Source: CAD feature listing. Evaluate the final solid. Frame: model axes, mm. Face numbers are marked on the shaded views. Give positions to 0.01 mm unless a question says otherwise; leave off trailing zeros. Write item = value, one per line.
from build123d import *

# Parameters (mm, degrees)
SKETCH_1_R          = 15
SKETCH_1_R_2        = 1.45
SKETCH_1_R_3        = 1.5
EXTRUDE_1_DEPTH     = 8
SKETCH_2_R          = 1.45
SKETCH_2_R_2        = 1.5
EXTRUDE_2_DEPTH     = 7
SKETCH_3_R          = 1.45
CUT_EXTRUDE_1_DEPTH = 8
SKETCH_4_R          = 1.45
CUT_EXTRUDE_2_DEPTH = 8
SKETCH_5_R          = 1.45
CUT_EXTRUDE_3_DEPTH = 8
SKETCH_6_R          = 1.45
CUT_EXTRUDE_4_DEPTH = 8
SKETCH_7_R          = 1.45
CUT_EXTRUDE_5_DEPTH = 8
SKETCH_8_R          = 1.5
CUT_EXTRUDE_6_DEPTH = 8
CHAMFER_1_SIZE      = 1.55


with BuildPart() as part:
    # 草图1 → 凸台-拉伸1 (new body)
    with BuildSketch(Plane(origin=(0, 0, 0), x_dir=(1, 0, 0), z_dir=(0, 1, 0))):
        Circle(SKETCH_1_R)
        with Locations((0, 12)):
            Circle(SKETCH_1_R_2, mode=Mode.SUBTRACT)
        with Locations((-10.392304845, -6)):
            Circle(SKETCH_1_R_2, mode=Mode.SUBTRACT)
        with Locations((10.392304845, -6)):
            Circle(SKETCH_1_R_2, mode=Mode.SUBTRACT)
        with Locations((-11.258330249, 6.5)):
            Circle(SKETCH_1_R_3, mode=Mode.SUBTRACT)
        with Locations((0, -13)):
            Circle(SKETCH_1_R_3, mode=Mode.SUBTRACT)
        with Locations((11.258330249, 6.5)):
            Circle(SKETCH_1_R_3, mode=Mode.SUBTRACT)
    extrude(amount=EXTRUDE_1_DEPTH)

    # 草图2 → 凸台-拉伸2 (add)
    with BuildSketch(Plane(origin=(0, 8, 0), x_dir=(1, 0, 0), z_dir=(0, 1, 0))):
        Polygon((0, 17.320508076), (-15, 8.660254038), (-15, -8.660254038), (0, -17.320508076), (15, -8.660254038), (15, 8.660254038), align=None)
        with Locations((0, 12)):
            Circle(SKETCH_2_R, mode=Mode.SUBTRACT)
        with Locations((-11.258330249, 6.5)):
            Circle(SKETCH_2_R_2, mode=Mode.SUBTRACT)
        with Locations((11.258330249, 6.5)):
            Circle(SKETCH_2_R_2, mode=Mode.SUBTRACT)
        with Locations((-10.392304845, -6)):
            Circle(SKETCH_2_R, mode=Mode.SUBTRACT)
        with Locations((0, -13)):
            Circle(SKETCH_2_R_2, mode=Mode.SUBTRACT)
        with Locations((10.392304845, -6)):
            Circle(SKETCH_2_R, mode=Mode.SUBTRACT)
    extrude(amount=-EXTRUDE_2_DEPTH)

    # 草图3 → 切除-拉伸1 (cut)
    with BuildSketch(Plane(origin=(7.5, 0, 12.990381057), x_dir=(0.866025404, 0, -0.5), z_dir=(0.5, 0, 0.866025404))):
        with Locations((0, 4.5)):
            Circle(SKETCH_3_R)
    extrude(amount=-CUT_EXTRUDE_1_DEPTH, mode=Mode.SUBTRACT)

    # 草图4 → 切除-拉伸2 (cut)
    with BuildSketch(Plane(origin=(-7.5, 0, 12.990381057), x_dir=(0.866025404, 0, 0.5), z_dir=(-0.5, 0, 0.866025404))):
        with Locations((0, 4.5)):
            Circle(SKETCH_4_R)
    extrude(amount=-CUT_EXTRUDE_2_DEPTH, mode=Mode.SUBTRACT)

    # 草图5 → 切除-拉伸3 (cut)
    with BuildSketch(Plane.ZY.offset(15)):
        with Locations((0, 4.5)):
            Circle(SKETCH_5_R)
    extrude(amount=-CUT_EXTRUDE_3_DEPTH, mode=Mode.SUBTRACT)

    # 草图6 → 切除-拉伸4 (cut)
    with BuildSketch(Plane(origin=(15, 0, 0), x_dir=(0, 0, -1), z_dir=(1, 0, 0))):
        with Locations((0, 4.5)):
            Circle(SKETCH_6_R)
    extrude(amount=-CUT_EXTRUDE_4_DEPTH, mode=Mode.SUBTRACT)

    # 草图7 → 切除-拉伸5 (cut)
    with BuildSketch(Plane(origin=(7.5, 0, -12.990381057), x_dir=(-0.866025404, 0, -0.5), z_dir=(0.5, 0, -0.866025404))):
        with Locations((0, 4.5)):
            Circle(SKETCH_7_R)
    extrude(amount=-CUT_EXTRUDE_5_DEPTH, mode=Mode.SUBTRACT)

    # 草图8 → 切除-拉伸6 (cut)
    with BuildSketch(Plane(origin=(-7.5, 0, -12.990381057), x_dir=(-0.866025404, 0, 0.5), z_dir=(-0.5, 0, -0.866025404))):
        with Locations((0, 4.5)):
            Circle(SKETCH_8_R)
    extrude(amount=-CUT_EXTRUDE_6_DEPTH, mode=Mode.SUBTRACT)

    # 倒角1
    chamfer_1_edges = [part.edges().sort_by_distance(p)[0] for p in [
        (8.942304845, 8, 6),
        (-1.45, 8, -12),
        (-11.842304845, 8, 6),
    ]]
    chamfer(chamfer_1_edges, length=CHAMFER_1_SIZE)


solid = part.part
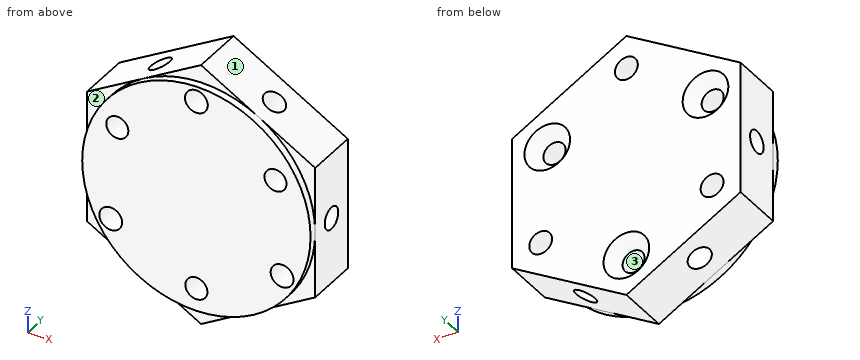
1. Pull-direction query (Z, two-part tool) for the marked faces 1, 2 and 3; classes: +Z half, -Z half, draft (parallel to the pull), parting line (faces both ways), or undercut.
Derived:
face_1 = +Z half
face_2 = draft
face_3 = undercut
2. Cut plane A-A, the plane z = 6. Count the separate pieces of the cut face and the enclosed holes in it, then the cut area to 3 significant figures.
Derived:
separate_pieces = 3
enclosed_holes = 2
area = 179 mm²
3. First-contact query: pin 1 Ø1 at (x, y) = (-4, 5.5) entering from -Z; pin 2 Ø3 at (x, y) = (0, 5.5) entering from +Z; pin 3 Ø1 at (x, y) = (1.5, 2.5) entering from -Z. Flat tips, straight axial feed; report the tip coordinate or a pass-through.
Derived:
pin_1 = -15.3
pin_2 = 17.32
pin_3 = -16.74
4. Material intervals for probe 1 along Z at (x, y) = (0, 5.75); probe 2 along Z at (x, y) = (0.5, 4.25); probe 3 along X at (y, z) = (4.75, 5.5), sorted ascending. Write a range as from..to.
Derived:
probe_1 = -17.32..-13.45, -10.55..11.5, 14.5..17.32
probe_2 = -17.03..-13.36, -10.64..11.59, 14.41..17.03
probe_3 = -15..-11.75, -9.03..-4.82, -4.47..4.47, 4.82..9.03, 11.75..15
